Answer from the drawing. Dimensions are ordinates in mm from the lowest x, y and z of the part. A direction names the side the tool comes from. Coordinates: 2 decimals unless noted, no trailing zeros. Loops run counter-clockwise (first coordinate to the right, second up) from the corner with the lowest first, then second, coordinate; pieces in that order, holes last.
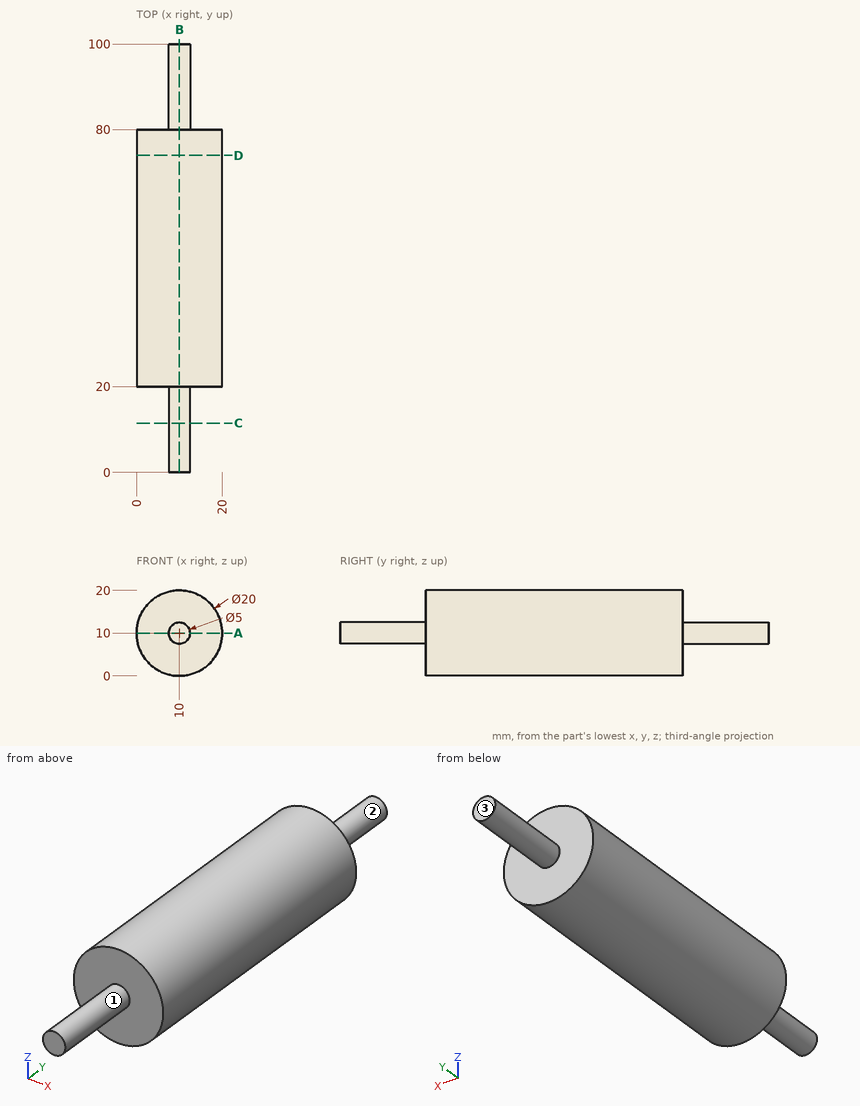
Item 1: A cutting plane is placed at D-D on y = 74. Determine the outline of the cut face in (x, z), then the cut area to 3 significant figures.
Numbers:
outline: circle Ø20 at (10, 10)
area: 314 mm2
Item 2: A cutting plane is placed at B-B on x = 10. Determine the outline of the cut face in (y, z).
Numbers:
outline: (0, 7.5) - (20, 7.5) - (20, 0) - (80, 0) - (80, 7.5) - (100, 7.5) - (100, 12.5) - (80, 12.5) - (80, 20) - (20, 20) - (20, 12.5) - (0, 12.5) - close
Item 3: A cutting plane is placed at C-C on y = 11.5. Determine the outline of the cut face in (x, z), then the cut area to 3 significant figures.
Numbers:
outline: circle Ø5 at (10, 10)
area: 19.6 mm2
Item 4: A cutting plane is placed at A-A on z = 10. Determine the outline of the cut face in (x, y).
Numbers:
outline: (0, 20) - (7.5, 20) - (7.5, 0) - (12.5, 0) - (12.5, 20) - (20, 20) - (20, 80) - (12.5, 80) - (12.5, 100) - (7.5, 100) - (7.5, 80) - (0, 80) - close
Item 5: Find the intervals of material crossed by line 1 along Y through (x, z) = (18.75, 5.25); line 2 along X through (y, z) = (77.5, 3.75); line 3 along X through (y, z) = (61, 2.5), in increasing order.
Numbers:
line 1: y = 20 to 80
line 2: x = 2.19 to 17.81
line 3: x = 3.39 to 16.61
Item 6: Given pin 1 (10 mm diameter, centred on x = 17, y = 74.5, fed in from +Z); pin 2 (6 mm diameter, centred on x = 4, z = 7.5, fed in from +Y); pin 3 (2 mm diameter, centred on x = 8, z = 3.5, fed in from -Y); pin 4 (4 mm diameter, centred on x = 15, y = 17.5, fed in from +Z), each flat-ended and moving along its own axis, determine where each tip first touches the part or whether it passes through.
Numbers:
pin 1: stops at z = 19.8
pin 2: stops at y = 80
pin 3: stops at y = 20
pin 4: passes through
Item 7: Which of the six approach directions +Z, -Z, +X, -X, +Y, -Y give full straight-line access (tool end or side, diameter ignored) to the marked faces 1, 2 and 3?
Numbers:
face 1: -Y
face 2: +Y
face 3: +Z, -Z, +X, -X, +Y
